Read the model definition and answer for the solid it produces. Units are mm, in the model's axes. Face numbers are marked on the shaded views. A direction names the side the tool comes from. Coordinates: 2 decimals unless noted, no trailing zeros. Order: outer loops, then holes, each group sorted by start corner. A loop starts at its lowest first (then second) coordinate and runs counter-clockwise, first axis right, second up. Notation, with made-up numbers: M 84,2.5 L 142,2.5 A23 ccw 142,34.5 Z; hole C -8.5,-19.5 d5. An arc over 180 degrees is marked long. Use a Markdown table: item, result. Add a question column.
1) Each of these flat-tipped pins is pushed along its axis until it touches: pin 1 Ø1.5 at (x, z) = (-1, 0.5) entering from +Y; pin 2 Ø13.5 at (x, z) = (0, 0) entering from +Y; pin 3 Ø0.6 at (y, z) = (9, 4.5) entering from +X; pin 4 Ø2.5 at (x, y) = (0, 6.91) entering from +Z. Where does it stop, or does it pass through?
2) Find the intervals of material crossed by probe 1 along X at (y, z) = (1.45, 0); probe 2 along X at (y, z) = (-1.5, 0); probe 3 along Y at (x, z) = (0, 6.5), in increasing order. Write a range as [from, to].
3) For the marked faces 1 and 2, determine the directions among +Z, -Z, +X, -X, +Y, -Y from which every point of the face is accessible in a straight line to the end or side of a thin tool.
4) The mould has two halves that part along Z. Classify the marked faces 3, 4 and 5: released by +Z, released by -Z, zero draft, split by the parting line, or undercut.
5) Find section A-A on y = 1.25. Write down the section's boundary in (x, z), plus the area to 3 significant figures.
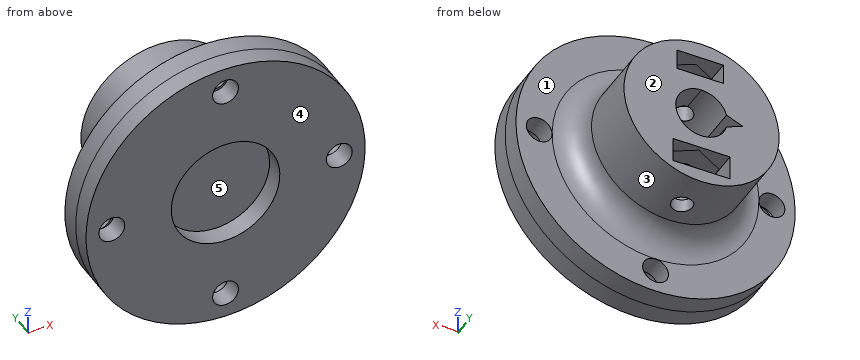
from build123d import *

# Parameters (mm, degrees)
SKETCH1_R               = 13.5
SKETCH1_R_2             = 1.25
BOSS_EXTRUDE2_DEPTH     = 2
SKETCH2_R               = 7.5
BOSS_EXTRUDE3_DEPTH     = 8.5
SKETCH4_R               = 2.5
CUT_EXTRUDE1_DEPTH      = 7.5
CUT_EXTRUDE2_DEPTH      = 7.5
CUT_EXTRUDE2_DEPTH_BACK = 11.75
SKETCH5_R               = 1
BOSS_EXTRUDE5_START     = 1.9
SKETCH7_R               = 13.5
SKETCH7_R_2             = 5.25
BOSS_EXTRUDE5_DEPTH     = 1.9
CUT_EXTRUDE3_DEPTH      = 8
FILLET1_R               = 2.5
SKETCH12_R              = 0.00537481
SKETCH12_R_2            = 0.008144056
SKETCH12_R_3            = 1.25
SKETCH12_R_4            = 0.012822725
CUT_EXTRUDE4_DEPTH      = 10
CIRPATTERN1_COUNT       = 4
SKETCH13_W              = 5.5
SKETCH13_H              = 2.4
SKETCH13_W_2            = 4.5
SKETCH13_H_2            = 2
CUT_EXTRUDE5_DEPTH      = 4
CUT_EXTRUDE6_DEPTH      = 2.4
CUT_EXTRUDE7_DEPTH      = 2


with BuildPart() as part:
    # Sketch1 → Boss-Extrude2 (new body)
    with BuildSketch(Plane(origin=(0, 0, 0), x_dir=(1, 0, 0), z_dir=(0, 1, 0))):
        with Locations(Location((0, 0, 0), (0, 0, 270))):
            Circle(SKETCH1_R)
        with Locations(Location((11.25, 0, 0), (0, 0, 270))):
            Circle(SKETCH1_R_2, mode=Mode.SUBTRACT)
        with Locations(Location((0, -11.25, 0), (0, 0, 270))):
            Circle(SKETCH1_R_2, mode=Mode.SUBTRACT)
        with Locations(Location((-11.25, 0, 0), (0, 0, 270))):
            Circle(SKETCH1_R_2, mode=Mode.SUBTRACT)
        with Locations(Location((0, 11.25, 0), (0, 0, 270))):
            Circle(SKETCH1_R_2, mode=Mode.SUBTRACT)
    extrude(amount=BOSS_EXTRUDE2_DEPTH)

    # Sketch2 → Boss-Extrude3 (add)
    with BuildSketch(Plane(origin=(0, 2, 0), x_dir=(1, 0, 0), z_dir=(0, 1, 0))):
        with Locations(Location((0, 0, 0), (0, 0, 270))):
            Circle(SKETCH2_R)
    extrude(amount=BOSS_EXTRUDE3_DEPTH)

    # Sketch4 → Cut-Extrude1 (cut)
    with BuildSketch(Plane(origin=(0, 10.5, 0), x_dir=(1, 0, 0), z_dir=(0, 1, 0))):
        with Locations(Location((0, 0, 0), (0, 0, 270))):
            Circle(SKETCH4_R)
    extrude(amount=-CUT_EXTRUDE1_DEPTH, mode=Mode.SUBTRACT)

    # Sketch5 → Cut-Extrude2 (cut, two sides: drawn at the far end of the back side and taken through both)
    with BuildSketch(Plane.XY.offset(-CUT_EXTRUDE2_DEPTH_BACK)):
        with Locations(Location((0, 6.914506731, 0), (0, 0, 180))):
            Circle(SKETCH5_R)
    extrude(amount=CUT_EXTRUDE2_DEPTH + CUT_EXTRUDE2_DEPTH_BACK, mode=Mode.SUBTRACT)

    # Sketch7 → Boss-Extrude5 (add)
    with BuildSketch(Plane.XZ.offset(BOSS_EXTRUDE5_START)):
        with Locations(Location((0, 0, 0), (0, 0, 270))):
            Circle(SKETCH7_R)
        with Locations(Location((0, 0, 0), (0, 0, 90))):
            Circle(SKETCH7_R_2, mode=Mode.SUBTRACT)
    extrude(amount=-BOSS_EXTRUDE5_DEPTH)

    # Sketch9 → Cut-Extrude3 (cut)
    with BuildSketch(Plane(origin=(0, 10.5, 0), x_dir=(1, 0, 0), z_dir=(0, 1, 0))):
        Polygon((-2.414753661, -0.64727487), (-2.414753661, 0.64727487), (-3.984419716, 0), align=None)
    extrude(amount=-CUT_EXTRUDE3_DEPTH, mode=Mode.SUBTRACT)

    # Fillet1
    fillet1_edges = [part.edges().sort_by_distance(p)[0] for p in [
        (0, 2, -7.5),
    ]]
    fillet(fillet1_edges, radius=FILLET1_R - 0.0001)  # a hair under: the kernel refuses the full size

    # Sketch12 → Cut-Extrude4 (cut)
    with BuildSketch(Plane(origin=(0, 0, 0), x_dir=(1, 0, 0), z_dir=(0, 1, 0))):
        with Locations(Location((-0.239113034, -10.028559531, 0), (0, 0, 101.087404696))):
            Circle(SKETCH12_R)
        with Locations(Location((-1.014615915, 11.966073133, 0), (0, 0, 144.78716899))):
            Circle(SKETCH12_R_2)
        with Locations(Location((-11, 0, 0), (0, 0, 264.260829523))):
            Circle(SKETCH12_R_3)
        with Locations(Location((10.492985163, 0.978537759, 0), (0, 0, 127.726196418))):
            Circle(SKETCH12_R_4)
    cut_extrude4 = extrude(amount=-CUT_EXTRUDE4_DEPTH, mode=Mode.SUBTRACT)

    # CirPattern1: Cut-Extrude4 ×4 about axis
    cirpattern1_axis = Axis((0, 0, 0), (0, 1, 0))
    for i in range(1, CIRPATTERN1_COUNT):
        add(cut_extrude4.rotate(cirpattern1_axis, i * 360 / CIRPATTERN1_COUNT), mode=Mode.SUBTRACT)

    # Sketch13 → Cut-Extrude5 (cut)
    with BuildSketch(Plane(origin=(0, 10.5, 0), x_dir=(1, 0, 0), z_dir=(0, 1, 0))):
        with Locations((0, 5)):
            Rectangle(SKETCH13_W, SKETCH13_H)
        with Locations((0.141735204, -5)):
            Rectangle(SKETCH13_W_2, SKETCH13_H_2)
    extrude(amount=-CUT_EXTRUDE5_DEPTH, mode=Mode.SUBTRACT)

    # Sketch14 → Cut-Extrude6 (cut)
    with BuildSketch(Plane(origin=(0, 0, -3.8), x_dir=(-1, 0, 0), z_dir=(0, 0, -1))):
        Polygon((2.721817224, 8.550063007), (-0.055524673, 10.089447729), (-2.777341897, 8.453891453), (-2.721817224, 5.278950455), (0.055524673, 3.739565732), (2.777341897, 5.375122009), align=None)
    extrude(amount=CUT_EXTRUDE6_DEPTH, mode=Mode.SUBTRACT)

    # Sketch15 → Cut-Extrude7 (cut)
    with BuildSketch(Plane.XY.offset(4)):
        Polygon((2.25, 8.213544837), (0, 9.512582942), (-2.25, 8.213544837), (-2.25, 5.615468625), (0, 4.31643052), (2.25, 5.615468625), align=None)
    extrude(amount=CUT_EXTRUDE7_DEPTH, mode=Mode.SUBTRACT)


solid = part.part
Check result:
| question | item | result |
|---|---|---|
| 1 | pin 1 | stops at y = 3 |
| 1 | pin 2 | stops at y = 10.5 |
| 1 | pin 3 | stops at x = 6.21 |
| 1 | pin 4 | stops at z = 7.5 |
| 2 | probe 1 | x = [-13.5, -12.5], [-10, 10], [12.5, 13.5] |
| 2 | probe 2 | x = [-13.5, -12.25], [-9.75, -5.25], [5.25, 9.75], [12.25, 13.5] |
| 2 | probe 3 | y = [-1.9, 5.91], [7.91, 10.5] |
| 3 | face 1 | +Y |
| 3 | face 2 | +Z, -Z, +X, -X, +Y |
| 4 | face 3 | split by the parting line |
| 4 | face 4 | zero draft |
| 4 | face 5 | undercut |
| 5 | outline | C 0,0 d27; hole C -11.25,0 d2.5; hole C 0,-11.25 d2.5; hole C 0,11.25 d2.5; hole C 11.25,0 d2.5 |
| 5 | area | 553 mm2 |
